Design review of the part built by this model. Coordinates are the model's own, in mm. Face numbers are marked on the shaded views. Coordinates: 2 decimals unless noted, no trailing zeros. Loops run counter-clockwise (first coordinate to the right, second up) from the corner with the lowest first, then second, coordinate; pieces in that order, holes last. Notation, with made-up numbers: M -7.75,42 L 33.25,42 A24 ccw 33.25,52 Z; hole C -14,15.5 d2. An arc over 180 degrees is marked long. Answer as a JSON object with one key per item and string values. Group by question number.
1. Draft analysis for pull direction X (two halves, no side actions). For the marked faces 1 and 2, state which applies: +X half, -X half, draft (parallel to the pull), parting line (faces both ways), or undercut.
2. Insertion check: pin 1 (6.5 mm diameter, centred on x = 27.5, z = -68, fed in from -Y); pin 2 (1 mm diameter, centred on x = 20.5, z = -57.5, fed in from +Y); pin 3 (4 mm diameter, centred on y = -3, z = -56.5, fed in from +X); pin 4 (1.5 mm diameter, centred on y = 0, z = -43.5, fed in from -X). Each pin has a flat end and moves straight along its axis. Give the tip position at first contact, or say it passes through.
3. To check wall thickness, follow probe 1 along X at (y, z) = (-2.5, -65); probe 2 along X at (y, z) = (-1, -69); probe 3 along X at (y, z) = (-2.75, -36.5). State the ranges of each line that lie inside material, in increasing order.
4. Consider section A-A (y = -1). State the section outline as (x, z) points.
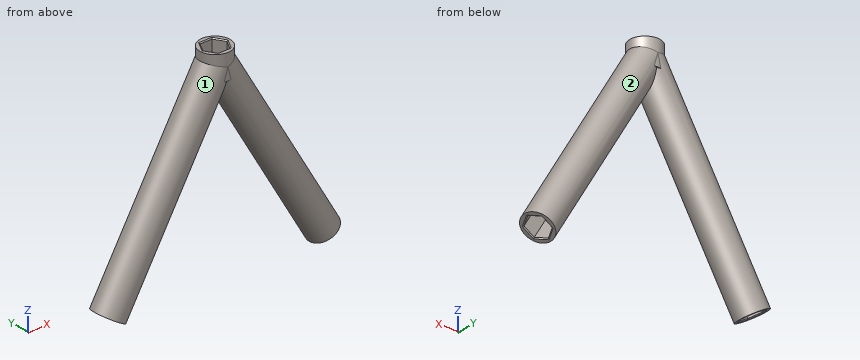
from build123d import *

# Parameters (mm, degrees)
SKETCH1_W          = 4
SKETCH1_H          = 6.6
CUT_EXTRUDE1_DEPTH = 6.6
CUT_EXTRUDE2_DEPTH = 6.6
CUT_EXTRUDE3_DEPTH = 6.6
CHAMFER1_SIZE      = 0.25


with BuildPart() as part:
    # Sketch1 → Revolve-Thin1 (revolve)
    with BuildSketch(Plane(origin=(0, 0, 0), x_dir=(1, 0, 0), z_dir=(0, 1, 0)), mode=Mode.PRIVATE) as revolve_thin1_sk:
        with Locations((-2, 20.8)):
            Rectangle(SKETCH1_W, SKETCH1_H)
    revolve(revolve_thin1_sk.sketch.rotate(Axis((0, 0, 0), (0, 0, -1)), 180), axis=Axis((0, 0, 0), (0, 0, -1)))

    # Sketch3 → Revolve-Thin2 (revolve)
    with BuildSketch(Plane(origin=(0, 0, 0), x_dir=(1, 0, 0), z_dir=(0, 1, 0)), mode=Mode.PRIVATE) as revolve_thin2_sk:
        Polygon((-28.888127, 69.742108), (0, 20.8), (3.444699, 22.833237), (-25.443428, 71.775345), align=None)
    revolve(revolve_thin2_sk.sketch.rotate(Axis((-28.888127, 0, -69.742108), (0.5083091776235522, 0, 0.8611746512430961)), 180), axis=Axis((-28.888127, 0, -69.742108), (0.5083091776235522, 0, 0.8611746512430961)))

    # Sketch4 → Revolve-Thin3 (revolve)
    with BuildSketch(Plane(origin=(0, 0, 0), x_dir=(1, 0, 0), z_dir=(0, 1, 0)), mode=Mode.PRIVATE) as revolve_thin3_sk:
        Polygon((0, 20.8), (28.888127, 69.742108), (25.443428, 71.775345), (-3.444699, 22.833237), align=None)
    revolve(revolve_thin3_sk.sketch.rotate(Axis((0, 0, -20.8), (0.5083091776235522, 0, -0.8611746512430961)), 180), axis=Axis((0, 0, -20.8), (0.5083091776235522, 0, -0.8611746512430961)))

    # Sketch5 → Cut-Extrude1 (cut)
    with BuildSketch(Plane(origin=(-37.993181, 0, -64.367841), x_dir=(-0.861174651243096, 0, 0.5083091776235522), z_dir=(-0.5083091776235522, 0, -0.861174651243096))):
        Polygon((-8.96491, 2.785), (-12.180751, 2.785), (-13.788672, 0), (-12.180751, -2.785), (-8.96491, -2.785), (-7.35699, 0), align=None)
    extrude(amount=-CUT_EXTRUDE1_DEPTH, mode=Mode.SUBTRACT)

    # Sketch6 → Cut-Extrude2 (cut)
    with BuildSketch(Plane.XY.offset(-17.5)):
        Polygon((1.60792, 2.785), (-1.60792, 2.785), (-3.215841, 0), (-1.60792, -2.785), (1.60792, -2.785), (3.215841, 0), align=None)
    extrude(amount=-CUT_EXTRUDE2_DEPTH, mode=Mode.SUBTRACT)

    # Sketch7 → Cut-Extrude3 (cut)
    with BuildSketch(Plane(origin=(37.993181, 0, -64.367841), x_dir=(-0.861174651243096, 0, -0.5083091776235522), z_dir=(0.5083091776235522, 0, -0.861174651243096))):
        Polygon((12.180751, 2.785), (8.96491, 2.785), (7.35699, 0), (8.96491, -2.785), (12.180751, -2.785), (13.788672, 0), align=None)
    extrude(amount=-CUT_EXTRUDE3_DEPTH, mode=Mode.SUBTRACT)

    # Chamfer1
    chamfer1_edges = [part.edges().sort_by_distance(p)[0] for p in [
        (-30.965178, 1.3925, -68.516127),
        (-28.888127, 2.785, -69.742108),
        (-26.811077, 1.3925, -70.968089),
        (-26.811077, -1.3925, -70.968089),
        (-28.888127, -2.785, -69.742108),
        (-30.965178, -1.3925, -68.516127),
        (2.411881, 1.3925, -17.5),
        (0, 2.785, -17.5),
        (-2.411881, 1.3925, -17.5),
        (-2.411881, -1.3925, -17.5),
        (0, -2.785, -17.5),
        (2.411881, -1.3925, -17.5),
        (26.811077, 1.3925, -70.968089),
        (28.888127, 2.785, -69.742108),
        (30.965178, 1.3925, -68.516127),
        (30.965178, -1.3925, -68.516127),
        (28.888127, -2.785, -69.742108),
        (26.811077, -1.3925, -70.968089),
    ]]
    chamfer(chamfer1_edges, length=CHAMFER1_SIZE)


solid = part.part
Findings below:
{
 "1": {"face 1": "undercut", "face 2": "undercut"},
 "2": {"pin 1": "stops at y = -4", "pin 2": "stops at y = 3.97", "pin 3": "stops at x = 26.17", "pin 4": "stops at x = -18.49"},
 "3": {"probe 1": "x = -29.71 to -28.15, -24.03 to -22.46, 22.46 to 24.03, 28.15 to 29.71", "probe 2": "x = -25.39 to -23.95, 23.95 to 25.39", "probe 3": "x = -12.64 to -5.89, 5.89 to 12.64"},
 "4": {"outline": "M -32.22,-67.77 L -31.41,-68.25 L -31.03,-68.19 L -27.81,-62.72 L -23.26,-65.4 L -26.49,-70.87 L -26.37,-71.23 L -25.55,-71.71 L 0,-28.42 L 25.55,-71.71 L 26.37,-71.23 L 26.49,-70.87 L 23.26,-65.4 L 27.81,-62.72 L 31.03,-68.19 L 31.41,-68.25 L 32.22,-67.77 L 3.87,-19.74 L 3.87,-17.5 L 2.93,-17.5 L 2.64,-17.75 L 2.64,-24.1 L -2.64,-24.1 L -2.64,-17.75 L -2.93,-17.5 L -3.87,-17.5 L -3.87,-19.74 Z"}
}
